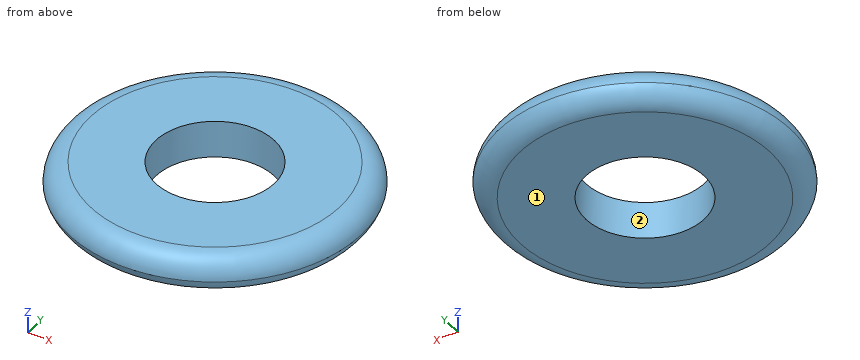
```python
from build123d import *

# Parameters (mm, degrees)
F0_R     = 27.5126478719
F0_R_2   = 11.2
F1_DEPTH = 7
F2_R     = 4


# Not quite as in the source:
# - a fillet or chamfer that OpenCascade refuses, or shapes differently, is made with other operations: its cross-section is extruded or revolved along the edge and cut away or added


with BuildPart() as f1:
    # F0 (on Top) → F1 (new body)
    with BuildSketch(Plane.XY):
        Circle(F0_R)
        Circle(F0_R_2, mode=Mode.SUBTRACT)
    extrude(amount=F1_DEPTH)

    # F2
    f2_edges = [f1.edges().sort_by_distance(p)[0] for p in [
        (-27.512648, 0, 7),
    ]]
    fillet(f2_edges, radius=F2_R)

    # F3: fillet of radius 4 on 1 edges, made by hand

    # F3_s1 → F3_t2 (revolve, cut)
    with BuildSketch(Plane.XZ):
        with BuildLine():
            ThreePointArc((27.5126478719, 3), (26.0891542684, 0.8377223398), (23.6396645256, 0))
            Line((23.6396645256, 0), (27.5126478719, 0))
            Line((27.5126478719, 0), (27.5126478719, 3))
        make_face()
    revolve(axis=Axis((0, 0, 0), (0, 0, 1)), mode=Mode.SUBTRACT)


solid = f1.part
```
CAD build for the part. Positions are in the model's coordinates, mm. Face numbers are marked on the shaded views. Round coordinates to 2 decimals unless told otherwise and drop trailing zeros. Order: outer loops, then holes, each group sorted by start corner. A loop starts at its lowest first (then second) coordinate and runs counter-clockwise, first axis right, second up.
Item 1: Pin check, flat tips, straight feed: pin 1 (3 mm diameter, centred on y = -17, z = 3.5, fed in from +X); pin 2 (3 mm diameter, centred on x = 16, z = 4.5, fed in from -Y). Stop position of each tip, or through.
Item 2: Saw through at A-A on y = 0. Write the cut outline in (x, z).
Item 3: Probe line 1 along Y through (x, z) = (-9, 1.75); line 2 along X through (y, z) = (-2.5, 1); line 3 along Y through (x, z) = (0, 4.5). List the from-to ranges inside material, lowest first.
Item 4: Mould opens along Y. For the marked faces 1 and 2 say: pulls with the +Y half, pulls with the -Y half, needs draft (parallel to the pull), parting line crosses it, or undercut.
Reported:
1. pin 1: stops at x = 22.71
1. pin 2: stops at y = -23.18
2. outline: (-27.51, 3) arc R4 ccw to (-23.64, 0) - (-11.2, 0) - (-11.2, 7) - (-23.51, 7) arc R4 ccw to start; (11.2, 0) - (23.64, 0) arc R4 ccw to (27.51, 3) arc R4 ccw to (23.51, 7) - (11.2, 7) - close
3. line 1: y = -25.4 to -6.67, 6.67 to 25.4
3. line 2: x = -26.17 to -10.92, 10.92 to 26.17
3. line 3: y = -27.22 to -11.2, 11.2 to 27.22
4. face 1: needs draft
4. face 2: undercut
